from build123d import *

# Parameters (mm, degrees)
SK_BASE_W  = 54
SK_BASE_H  = 20
BASE_DEPTH = 23
SK_HEAD_W  = 19
SK_HEAD_H  = 15


with BuildPart() as part:
    # SK_Base → Base (new, symmetric)
    with BuildSketch(Plane.XY):
        with Locations((0, 10)):
            Rectangle(SK_BASE_W, SK_BASE_H)
    extrude(amount=BASE_DEPTH, both=True)

    # SK_Head → Head (revolve)
    with BuildSketch(Plane.XY, mode=Mode.PRIVATE) as head_sk:
        with Locations((9.5, 27.5)):
            Rectangle(SK_HEAD_W, SK_HEAD_H)
    revolve(head_sk.sketch.rotate(Axis((0, 15, 0), (0, 1, 0)), 90), axis=Axis((0, 15, 0), (0, 1, 0)))


solid = part.part
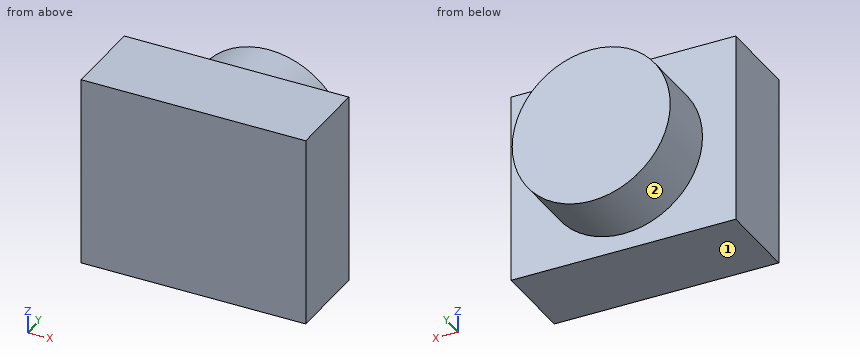
Design review of the part built by this model. Coordinates are the model's own, in mm. Face numbers are marked on the shaded views. A direction names the side the tool comes from. Coordinates: 2 decimals unless noted, no trailing zeros. Loops run counter-clockwise (first coordinate to the right, second up) from the corner with the lowest first, then second, coordinate; pieces in that order, holes last.
Item 1: For the marked faces 1 and 2, list the 3-axis set-ups (+Z, -Z, +X, -X, +Y, -Y) from which the entire face can be reached by the end or side of a thin tool; tool diameter is ignored.
Completed:
face 1: -Z, +X, -X, +Y, -Y
face 2: +Y
Item 2: Add section D-D (x = 20.5). Write out the cut boundary in (y, z).
Completed:
outline: (0, -23) - (20, -23) - (20, 23) - (0, 23) - close
Item 3: Add section B-B (x = 0). Write out the cut boundary in (y, z).
Completed:
outline: (0, -23) - (20, -23) - (20, -19) - (35, -19) - (35, 19) - (20, 19) - (20, 23) - (0, 23) - close
Item 4: Clearance check with flat-ended pins moving along their axes: pin 1 (1 mm diameter, centred on x = 11, z = 12.5, fed in from -Y); pin 2 (4 mm diameter, centred on x = -17, y = 25.5, fed in from -Z). State where each tip first meets the part, or that it passes through.
Completed:
pin 1: stops at y = 0
pin 2: stops at z = -11.66
Item 5: Add section C-C (y = 22). Write out the cut boundary in (x, z).
Completed:
outline: circle Ø38 at (0, 0)
Item 6: Add section A-A (z = 0). Write out the cut boundary in (x, y), and give its area (3 significant figures).
Completed:
outline: (-27, 0) - (27, 0) - (27, 20) - (19, 20) - (19, 35) - (-19, 35) - (-19, 20) - (-27, 20) - close
area: 1,650 mm2
Item 7: Wall thickness on L1, parallel to Y at x = 23, z = 11.5; L2, parallel to Z at x = -10, y = 25.5; L3, parallel to X at y = 29.5, z = -2.5: over which ranges is each line inside the solid? List them lowest first.
Completed:
L1: y = 0 to 20
L2: z = -16.16 to 16.16
L3: x = -18.83 to 18.83
